The figure shows three views and two pictorial views of one solid part (mm, origin at its lowest corner). Answer the questions. A direction names the side the tool comes from. Round coordinates to 2 decimals unless told otherwise and drop trailing zeros. Order: outer loops, then holes, each group sorted by start corner. A loop starts at its lowest first (then second) coordinate and runs counter-clockwise, first axis right, second up. Notation, with made-up numbers: (46.25, 38.25) - (68.25, 38.25) arc R20 cw to (68.25, 48.25) - close; hole circle Ø2 at (89.5, 65.25). An arc over 180 degrees is marked (long way). One line per item, written item: value. Start each with the question number.
1. A tool of negligible diameter and unlimited length cuts with its end or side. For the marked faces 1 and 2, from which of +Z, -Z, +X, -X, +Y, -Y can it reach the whole face along a straight path? Write none if from no direction.
2. A straight line is drawn through the part: line 1 (Y direction, x = 7.5, z = 20) (1 decimal). Find the intervals that lie inside material, in ascending order.
3. Section B-B, the plane z = 7.5 is taken. Give the vertices of the cut face in (x, y) (1 decimal), then the cut area to 3 significant figures.
4. Section C-C, the plane x = 11.5 is taken. Count the separate pieces of the cut face and the enclosed holes in it.
5. Flat-ended cylindrical pins translate along their axes: P1, Ø3, axis at x = 30.5, y = 15, coming from the -Z side (1 decimal); P2, Ø2.5, axis at x = 11.11, z = 8.72, coming from the +Y side; P3, Ø4.5, axis at x = 36.51, z = 21.42, coming from the +Y side (1 decimal). Find the tip coordinate at first contact, or state that the pin passes through.
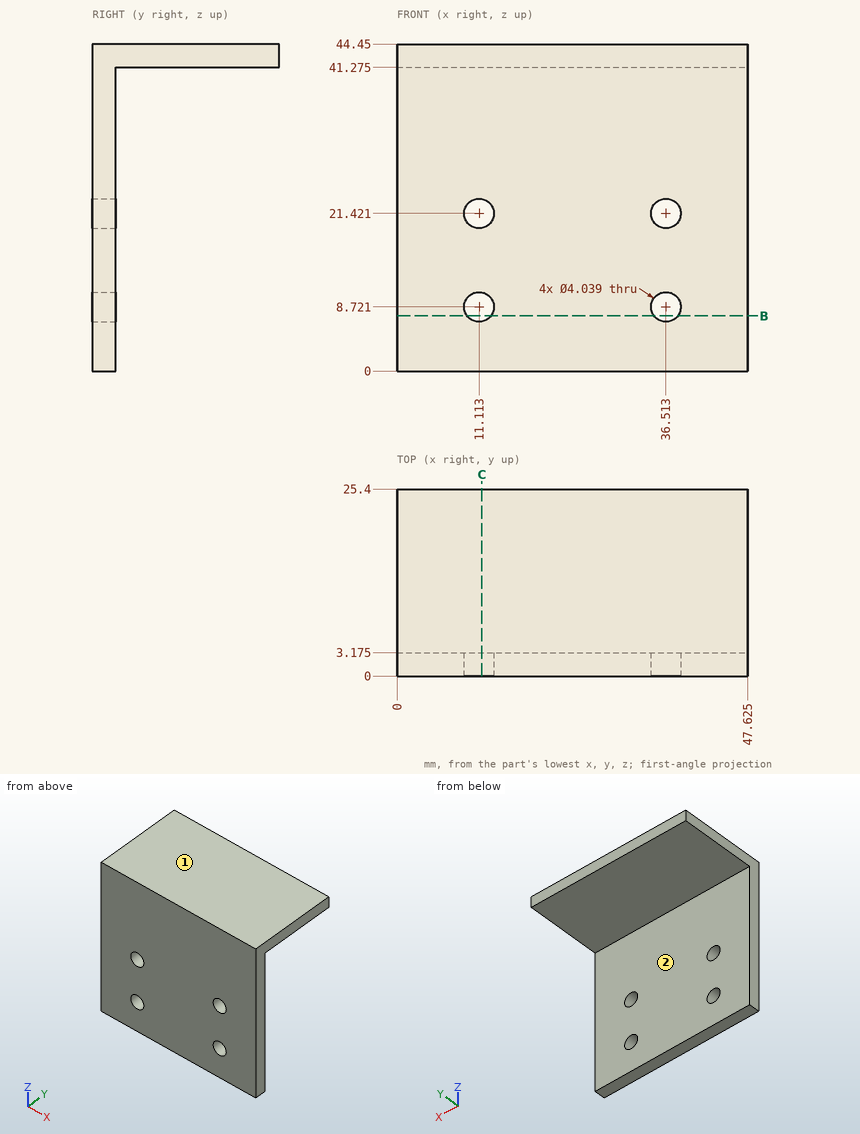
Answer list:
1. face 1: +Z, +X, -X, +Y, -Y
1. face 2: -Z, +X, -X, +Y
2. line 1: y = 0 to 3.2
3. outline: (0, 0) - (9.5, 0) - (9.5, 3.2) - (0, 3.2) - close; (12.7, 0) - (34.9, 0) - (34.9, 3.2) - (12.7, 3.2) - close; (38.1, 0) - (47.6, 0) - (47.6, 3.2) - (38.1, 3.2) - close
3. area: 131 mm²
4. separate pieces: 3
4. enclosed holes: 0
5. P1: stops at z = 41.3
5. P2: passes through
5. P3: stops at y = 3.2
